Source: CAD feature listing. Evaluate the final solid. Frame: model axes, mm. A direction names the side the tool comes from. Give positions to 0.01 mm unless a question says otherwise; leave off trailing zeros. Order: outer loops, then holes, each group sorted by start corner. A loop starts at its lowest first (then second) coordinate and runs counter-clockwise, first axis right, second up.
```python
from build123d import *

# Parameters (mm, degrees)
SALIENTE_EXTRUIR1_DEPTH = 3


with BuildPart() as part:
    # Croquis1 → Saliente-Extruir1 (new body)
    with BuildSketch(Plane.XY):
        Polygon((8.3, 21.5), (-7.5, 21.5), (-7.5, 18.5), (-50, 18.5), (-50, -18.5), (-35.7, -18.5), (-35.7, -21.5), (-20, -21.5), (-20, -18.5), (18.4, -18.5), (18.4, -21.5), (34.1, -21.5), (34.1, -18.5), (50, -18.5), (50, 18.5), (8.3, 18.5), align=None)
        with BuildLine():
            ThreePointArc((-48.7, 0.9), (-48.407106781, 1.607106781), (-47.7, 1.9))
            Line((-47.7, 1.9), (-39.7, 1.9))
            ThreePointArc((-39.7, 1.9), (-38.992893219, 1.607106781), (-38.7, 0.9))
            Line((-38.7, 0.9), (-38.7, -9.1))
            ThreePointArc((-38.7, -9.1), (-38.992893219, -9.807106781), (-39.7, -10.1))
            Line((-39.7, -10.1), (-47.7, -10.1))
            ThreePointArc((-47.7, -10.1), (-48.407106781, -9.807106781), (-48.7, -9.1))
            Line((-48.7, -9.1), (-48.7, 0.9))
        make_face(mode=Mode.SUBTRACT)
        with BuildLine():
            ThreePointArc((-13.8, -10.2), (-14.507106781, -10.492893219), (-14.8, -11.2))
            Line((-14.8, -11.2), (-14.8, -11.5))
            ThreePointArc((-14.8, -11.5), (-15.092893219, -12.207106781), (-15.8, -12.5))
            Line((-15.8, -12.5), (-36.3, -12.5))
            ThreePointArc((-36.3, -12.5), (-37.007106781, -12.207106781), (-37.3, -11.5))
            Line((-37.3, -11.5), (-37.3, 11.3))
            ThreePointArc((-37.3, 11.3), (-37.007106781, 12.007106781), (-36.3, 12.3))
            Line((-36.3, 12.3), (-15.8, 12.3))
            ThreePointArc((-15.8, 12.3), (-15.092893219, 12.007106781), (-14.8, 11.3))
            Line((-14.8, 11.3), (-14.8, 8.3))
            ThreePointArc((-14.8, 8.3), (-14.507106781, 7.592893219), (-13.8, 7.3))
            Line((-13.8, 7.3), (16.4, 7.3))
            ThreePointArc((16.4, 7.3), (17.107106781, 7.007106781), (17.4, 6.3))
            Line((17.4, 6.3), (17.4, 5.8))
            ThreePointArc((17.4, 5.8), (17.692893219, 5.092893219), (18.4, 4.8))
            Line((18.4, 4.8), (34.3, 4.8))
            ThreePointArc((34.3, 4.8), (35.007106781, 4.507106781), (35.3, 3.8))
            Line((35.3, 3.8), (35.3, -2.2))
            ThreePointArc((35.3, -2.2), (35.592893219, -2.907106781), (36.3, -3.2))
            Line((36.3, -3.2), (46.3, -3.2))
            ThreePointArc((46.3, -3.2), (47.007106781, -3.492893219), (47.3, -4.2))
            Line((47.3, -4.2), (47.3, -12.5))
            ThreePointArc((47.3, -12.5), (47.007106781, -13.207106781), (46.3, -13.5))
            Line((46.3, -13.5), (34.9, -13.5))
            ThreePointArc((34.9, -13.5), (34.192893219, -13.207106781), (33.9, -12.5))
            Line((33.9, -12.5), (33.9, -11.2))
            ThreePointArc((33.9, -11.2), (33.607106781, -10.492893219), (32.9, -10.2))
            Line((32.9, -10.2), (17.4, -10.2))
            Line((17.4, -10.2), (-13.8, -10.2))
        make_face(mode=Mode.SUBTRACT)
    extrude(amount=SALIENTE_EXTRUIR1_DEPTH)


solid = part.part
```
1) Pin query (flat end, axial travel): pin 1 (1.5 mm diameter, centred on y = -20, z = 1.5, fed in from +X); pin 2 (0.9 mm diameter, centred on y = 20, z = 2, fed in from -X); pin 3 (0.9 mm diameter, centred on x = 21.5, z = 1.5, fed in from +Y); pin 4 (12 mm diameter, centred on x = -34, y = 17, fed in from -Z). Return the tip coordinate at first contact, or that it passes through.
Report:
pin 1: stops at x = 34.1
pin 2: stops at x = -7.5
pin 3: stops at y = 18.5
pin 4: stops at z = 0
2) Material intervals for L1, parallel to X at y = -1.5, z = 1.4; L2, parallel to X at y = -11.5, z = 2.5; L3, parallel to Y at x = -18, z = 2.9, sorted ascending.
Report:
L1: x = -50 to -48.7, -38.7 to -37.3, 35.3 to 50
L2: x = -50 to -37.3, -14.8 to 33.9, 47.3 to 50
L3: y = -18.5 to -12.5, 12.3 to 18.5
3) Section query A-A, the plane x = 12.5. Return the cut outline in (y, z).
Report:
outline: (-18.5, 0) - (-10.2, 0) - (-10.2, 3) - (-18.5, 3) - close; (7.3, 0) - (18.5, 0) - (18.5, 3) - (7.3, 3) - close
4) Section query C-C, the plane x = -34. Return the cut outline in (y, z).
Report:
outline: (-21.5, 0) - (-12.5, 0) - (-12.5, 3) - (-21.5, 3) - close; (12.3, 0) - (18.5, 0) - (18.5, 3) - (12.3, 3) - close
5) Section query B-B, the plane y = -0.5. Return the cut outline in (x, z), and give its area (3 significant figures).
Report:
outline: (-50, 0) - (-48.7, 0) - (-48.7, 3) - (-50, 3) - close; (-38.7, 0) - (-37.3, 0) - (-37.3, 3) - (-38.7, 3) - close; (35.3, 0) - (50, 0) - (50, 3) - (35.3, 3) - close
area: 52.2 mm2
6) Reachability of faces 1 (the flat face through (29, 18.5, 1)), 2 (the flat face through (42, -18.5, 1)), 3 (the flat face through (-20, -20, 1)), 4 (the flat face through (35.3, 1, 1)) from +Z, -Z, +X, -X, +Y, -Y: full face, straight path, thin tool, end or side. Return the list, or none.
Report:
face 1: +Z, -Z, +X, +Y
face 2: +Z, -Z, +X, -Y
face 3: +Z, -Z, -Y
face 4: +Z, -Z
7) Draft query along X for faces 5 (the flat face through (-44, 1.9, 1)), 6 (the flat face through (-28, 18.5, 1)). Return one class per face: +X half, -X half, draft (parallel to the pull), parting line (faces both ways), or undercut.
Report:
face 5: undercut
face 6: draft
8) Section query D-D, the plane z = 1.35. Count the separate pieces of the cut face and the enclosed holes in it, and give its area (3 significant figures).
Report:
separate pieces: 1
enclosed holes: 2
area: 2,210 mm2
